from build123d import *

# Parameters (mm, degrees)
SKETCH_1_R          = 1.6
SKETCH_1_W          = 15
SKETCH_1_H          = 6
EXTRUDE_1_DEPTH     = 3
FILLET_1_R          = 2
FILLET_2_R          = 3
SKETCH_2_R          = 1.6
SKETCH_2_W          = 32
SKETCH_2_H          = 12.112345176
CUT_EXTRUDE_1_DEPTH = 44.829670316
FILLET_3_R          = 1


with BuildPart() as part:
    # 草图1 → 凸台-拉伸1 (new body)
    with BuildSketch(Plane.XY):
        Polygon((0, 0), (0, 26.8), (12, 26.8), (12, 29.8), (22, 29.8), (22, 26.8), (32, 26.8), (32, 0), align=None)
        with Locations((3, 17)):
            Circle(SKETCH_1_R, mode=Mode.SUBTRACT)
        with Locations((3, 10)):
            Circle(SKETCH_1_R, mode=Mode.SUBTRACT)
        with Locations((20.5, 7)):
            Rectangle(SKETCH_1_W, SKETCH_1_H, mode=Mode.SUBTRACT)
        with Locations((20.5, 18)):
            Rectangle(SKETCH_1_W, SKETCH_1_H, mode=Mode.SUBTRACT)
    extrude(amount=EXTRUDE_1_DEPTH)

    # 圆角1
    fillet_1_edges = [part.edges().sort_by_distance(p)[0] for p in [
        (13, 10, 1.5),
        (13, 4, 1.5),
        (28, 4, 1.5),
        (28, 10, 1.5),
        (13, 21, 1.5),
        (13, 15, 1.5),
        (28, 15, 1.5),
        (28, 21, 1.5),
    ]]
    fillet(fillet_1_edges, radius=FILLET_1_R)

    # 圆角2
    fillet_2_edges = [part.edges().sort_by_distance(p)[0] for p in [
        (0, 0, 1.5),
        (32, 0, 1.5),
    ]]
    fillet(fillet_2_edges, radius=FILLET_2_R)

    # 草图2 → 切除-拉伸1 (cut, through all)
    with BuildSketch(Plane.XY.offset(3)):
        with Locations((29.2, 13.5)):
            Circle(SKETCH_2_R)
        with Locations((16, 25.556172588)):
            Rectangle(SKETCH_2_W, SKETCH_2_H)
        with Locations((16, 1.443827412)):
            Rectangle(SKETCH_2_W, SKETCH_2_H)
    extrude(amount=-CUT_EXTRUDE_1_DEPTH, mode=Mode.SUBTRACT)

    # 圆角3
    fillet_3_edges = [part.edges().sort_by_distance(p)[0] for p in [
        (28, 7.5, 1.5),
        (13, 7.5, 1.5),
        (13.063508327, 19.5, 1.5),
        (27.936491673, 19.5, 1.5),
    ]]
    fillet(fillet_3_edges, radius=FILLET_3_R)


solid = part.part
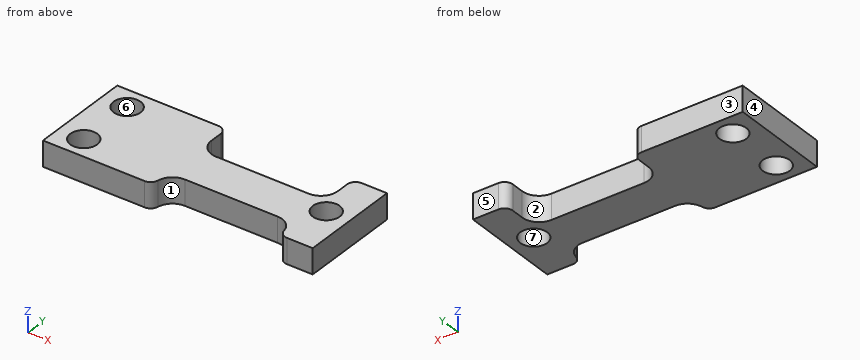
Work out the finished part from the listing and answer in its coordinate system (mm). Face numbers are marked on the shaded views. A direction names the side the tool comes from. Give positions to 0.01 mm unless a question says otherwise; leave off trailing zeros. Loops run counter-clockwise (first coordinate to the right, second up) from the corner with the lowest first, then second, coordinate; pieces in that order, holes last. Notation, with made-up numbers: (75, -25) -> (120, -25) arc R11 ccw to (120, -18) -> close; hole circle Ø9 at (61.5, -5). An arc over 180 degrees is marked (long way). Use a Markdown table: item, result. Add a question column.
1) For a pull along Y with two mould halves and no side action, classify the marked faces 4, 5, 6 and 7 as +Y half, -Y half, draft (parallel to the pull), parting line (faces both ways), or undercut.
2) Consider line 1 along Y through (x, z) = (3, 1.3); line 2 along Y through (x, z) = (29.2, 1.75); line 3 along X through (y, z) = (17.25, 1.05). Determine where each line is inside the solid, lowest interval first.
3) The part is cut by section C-C, the plane x = 20. Determine the outline of the cut face in (y, z), plus the area to 3 significant figures.
4) The part is cut by section D-D, the plane y = 12.25. Determine the outline of the cut face in (x, z), plus the area to 3 significant figures.
5) The part is cut by section A-A, the plane y = 13.5. Determine the outline of the cut face in (x, z), plus the area to 3 significant figures.
6) The part is cut by section B-B, the plane z = 0.75. Count the separate pieces of the cut face and the enclosed holes in it, plus the area to 3 significant figures.
7) This flat-tipped pin is pushed along its axis until it touches: P1, Ø0.9, axis at x = 20, z = 2, coming from the -Y side. Where does it stop, or does it pass through?
8) Which of the six approach directions +Z, -Z, +X, -X, +Y, -Y give full straight-line access (tool end or side, diameter ignored) to the marked faces 1, 2 and 3?
Reported:
| question | item | result |
|---|---|---|
| 1 | face 4 | draft |
| 1 | face 5 | +Y half |
| 1 | face 6 | undercut |
| 1 | face 7 | undercut |
| 2 | line 1 | y = 7.5 to 8.4, 11.6 to 15.4, 18.6 to 19.5 |
| 2 | line 2 | y = 7.5 to 11.9, 15.1 to 19.5 |
| 2 | line 3 | x = 0 to 1.42, 4.58 to 13, 28 to 32 |
| 3 | outline | (10, 0) -> (15, 0) -> (15, 3) -> (10, 3) -> close |
| 3 | area | 15.0 mm^2 |
| 4 | outline | (0, 0) -> (28.2, 0) -> (28.2, 3) -> (0, 3) -> close; (30.2, 0) -> (32, 0) -> (32, 3) -> (30.2, 3) -> close |
| 4 | area | 90.0 mm^2 |
| 5 | outline | (0, 0) -> (27.6, 0) -> (27.6, 3) -> (0, 3) -> close; (30.8, 0) -> (32, 0) -> (32, 3) -> (30.8, 3) -> close |
| 5 | area | 86.4 mm^2 |
| 6 | separate pieces | 1 |
| 6 | enclosed holes | 3 |
| 6 | area | 258 mm^2 |
| 7 | P1 | stops at y = 10 |
| 8 | face 1 | +Z, -Z, -Y |
| 8 | face 2 | +Z, -Z, +Y |
| 8 | face 3 | +Z, -Z, +X, -X, +Y |
